Could you check a few things on this model? Use its own coordinates, in mm. Face numbers are marked on the shaded views. A direction names the side the tool comes from. Round coordinates to 2 decimals unless told otherwise and drop trailing zeros. Loops run counter-clockwise (first coordinate to the right, second up) from the corner with the lowest first, then second, coordinate; pieces in that order, holes last.
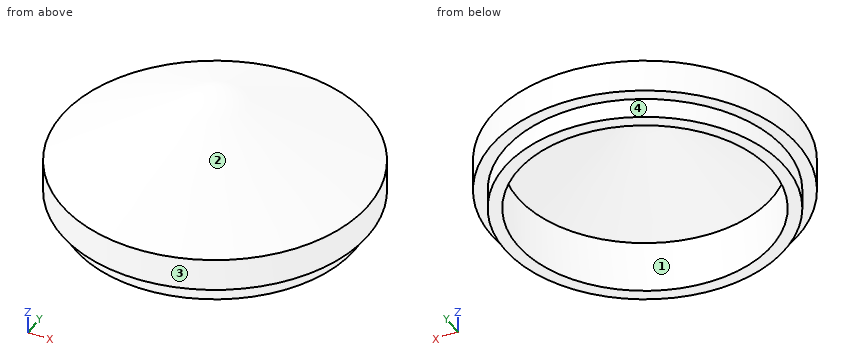
from build123d import *

# Parameters (mm, degrees)
F0_R     = 47
F1_DEPTH = 16
F2_R     = 39
F3_DEPTH = 16
F4_R     = 47
F4_R_2   = 43
F5_DEPTH = 6


with BuildPart() as f1:
    # F0 (on Top) → F1 (new body)
    with BuildSketch(Plane.XY):
        Circle(F0_R)
    extrude(amount=F1_DEPTH)

    # F2 (on face) → F3 (cut)
    with BuildSketch(Plane(origin=(0, 0, 0), x_dir=(1, 0, 0), z_dir=(0, 0, -1))):
        Circle(F2_R)
    extrude(amount=-F3_DEPTH, mode=Mode.SUBTRACT)

    # F4 (on face) → F5 (cut)
    with BuildSketch(Plane(origin=(0, 0, 0), x_dir=(1, 0, 0), z_dir=(0, 0, -1))):
        Circle(F4_R)
        Circle(F4_R_2, mode=Mode.SUBTRACT)
    extrude(amount=-F5_DEPTH, mode=Mode.SUBTRACT)

    # F7 (on Front) → F8 (revolve)
    with BuildSketch(Plane.XZ):
        Polygon((-39, 16), (0, 36.744681), (0, 41), (-47, 16), align=None)
    revolve(axis=Axis((0, 0, 12.147951), (0, 0, 1)))


solid = f1.part
Item 1: We'd pull the mould along Y, two halves only. Please class the marked faces 1 and 2: released by +Y, released by -Y, zero draft, split by the parting line, or undercut.
Results list:
face 1: undercut
face 2: split by the parting line
Item 2: For the marked faces 3 and 4, which set-ups out of +Z, -Z, +X, -X, +Y, -Y let a thin tool reach every point of the face, with its end or its side?
Results list:
face 3: +Z, -Z
face 4: -Z
Item 3: If I drill on line 1 along Y through (x, z) = (0, 3); line 2 along X through (y, z) = (0, 9), over which ranges is the centre line in solid material (lowest first)?
Results list:
line 1: y = -43 to -39, 39 to 43
line 2: x = -47 to -39, 39 to 47
Item 4: If we section it at A-A, the plane z = 32: Please give me the cut outline in (x, y).
Results list:
outline: circle Ø33.84 at (0, 0); hole circle Ø17.84 at (0, 0)
Item 5: Will these pins go through, and if not, where does the flat tip stop? pin 1 (10 mm diameter, centred on x = 22.5, z = 18, fed in from +Y); pin 2 (1.5 mm diameter, centred on x = 30, y = -11, fed in from -Z); pin 3 (3 mm diameter, centred on y = 32.5, z = 8.5, fed in from +X); pin 4 (2 mm diameter, centred on y = -17, z = 34, fed in from -X).
Results list:
pin 1: stops at y = 43.45
pin 2: stops at z = 19.35
pin 3: stops at x = 35.33
pin 4: passes through
Item 6: If we section it at B-B, the plane z = 38.5: Please give me the cut outline in (x, y).
Results list:
outline: circle Ø9.4 at (0, 0)
